Autodesk Inventor part; units mm, degrees
ref_plane "YZ Plane" through (0, 0, 0) normal (1, 0, 0) x (0, 1, 0)
ref_plane "XZ Plane" through (0, 0, 0) normal (0, 1, 0) x (-1, 0, 0)
ref_plane "XY Plane" through (0, 0, 0) normal (0, 0, 1) x (1, 0, 0)
sketch "Sketch1" plane through (0, 0, 0) normal (0, 1, 0) x (-1, 0, 0)
  point P0 (0, 0)
sketch "Sketch2" plane through (0, 0, 0) normal (0, 1, 0) x (-1, 0, 0)
  line L0 (2.7724, 24.8182) -> (-3.2276, 24.8182)
  line L1 (2.7724, 24.8182) -> (2.7724, -20.1818)
  line L2 (-3.2276, 24.8182) -> (-3.2276, -20.1818)
  line L3 (-3.2276, -20.1818) -> (-1.0276, -20.1818)
  line L4 (2.7724, -20.1818) -> (0.5724, -20.1818)
  line L5 (-1.0276, -20.1818) -> (0.5724, -20.1818)
  point P0 (0, 0)
  dimension "d0" = 6
  dimension "d1" = 45
  dimension "d2" = 45
  dimension "d3" = 2.2
  dimension "d4" = 2.2
extrude "Extrusion1" add sketch "Sketch2" along normal blind 3
sketch "Sketch4" plane through (0, 0, 0) normal (0, -1, 0) x (1, 0, 0)
  line L0 (-2.7724, 24.8182) -> (3.2276, 24.8182)
  circle A0 centre (0.2276, 19.8001) radius 1.2121
  line L1 (-2.7724, -20.1818) -> (-2.7724, 24.8182)
  circle A1 centre (0.2276, -15.1638) radius 1.2121
  point P0 (0, 0)
extrude "Extrusion3" cut sketch "Sketch4" against normal blind 10.9375 contours A0
extrude "Extrusion4" cut sketch "Sketch4" against normal blind 10.6375 contours A1
properties part number "LInk1"
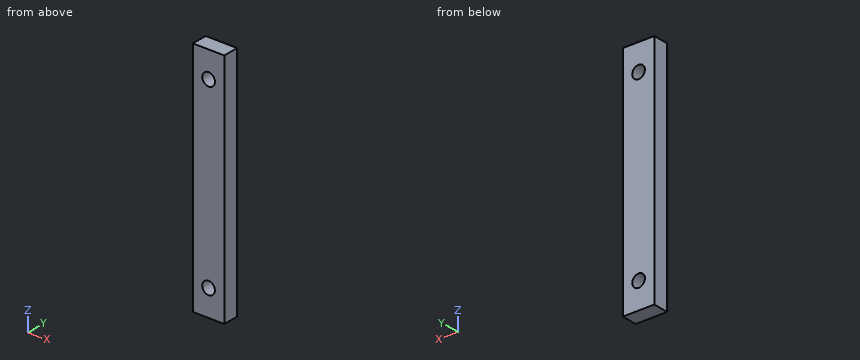
The model under review builds one solid part; all positions refer to its coordinate system, in mm. Give positions to 0.01 mm unless a question says otherwise; leave off trailing zeros. Loops run counter-clockwise (first coordinate to the right, second up) from the corner with the lowest first, then second, coordinate; pieces in that order, holes last. Notation, with made-up numbers: (69.5, -37) -> (116.5, -37) arc R20 cw to (116.5, -10) -> close; hole circle Ø7 at (6, -27). An arc over 180 degrees is marked (long way). Answer as a JSON object with one key per item and string values. Group by question number.
Q1. Take a section at A-A (x = 0.9). Write out the cut boundary in (y, z).
Q2. Wall thickness on line 1 along Z through (x, y) = (1.15, 2.3); line 2 along Z through (x, y) = (0.9, 2.55); line 3 along X through (y, z) = (2.7, 20): over which ranges is each line inside the solid? List them lowest first.
Q3. Take a section at B-B (y = 1.85). Write out the cut boundary in (x, z), plus the area to 3 significant figures.
Q4. Insertion check: pin 1 (3 mm diameter, centred on x = 0.5, z = -9.5, fed in from -Y); pin 2 (2 mm diameter, centred on x = 0.23, z = 19.8, fed in from -Y). Each pin has a flat end and moves straight along its axis. Give the tip position at first contact, or say it passes through.
Answer below:
{
 "1": {"outline": "(0, -20.18) -> (3, -20.18) -> (3, -16.17) -> (0, -16.17) -> close; (0, -14.16) -> (3, -14.16) -> (3, 18.79) -> (0, 18.79) -> close; (0, 20.81) -> (3, 20.81) -> (3, 24.82) -> (0, 24.82) -> close"},
 "2": {"line 1": "z = -20.18 to -15.95, -14.38 to 19.01, 20.59 to 24.82", "line 2": "z = -20.18 to -16.17, -14.16 to 18.79, 20.81 to 24.82", "line 3": "x = -2.77 to -0.97, 1.42 to 3.23"},
 "3": {"outline": "(-2.77, -20.18) -> (3.23, -20.18) -> (3.23, 24.82) -> (-2.77, 24.82) -> close; hole circle Ø2.42 at (0.23, -15.16); hole circle Ø2.42 at (0.23, 19.8)", "area": "261 mm2"},
 "4": {"pin 1": "stops at y = 0", "pin 2": "passes through"}
}
